```python
from build123d import *

# Parameters (mm, degrees)
F0_W     = 977.9
F0_H     = 38.1
F1_DEPTH = 19.05
F3_DEPTH = 25.4
F5_DEPTH = 25.4


with BuildPart() as f1:
    # F0 (on Front) → F1 (new body)
    with BuildSketch(Plane.XZ):
        with Locations((-488.95, 19.05)):
            Rectangle(F0_W, F0_H)
    extrude(amount=F1_DEPTH)

    # F2 (on face) → F3 (cut)
    with BuildSketch(Plane.XZ.offset(19.05)):
        Polygon((-971.181942, 0), (-977.9, 38.1), (-977.9, 0), align=None)
    extrude(amount=-F3_DEPTH, mode=Mode.SUBTRACT)

    # F4 (on face) → F5 (cut)
    with BuildSketch(Plane.XZ.offset(19.05)):
        Polygon((0, 0), (0, 38.1), (-6.718058, 0), align=None)
    extrude(amount=-F5_DEPTH, mode=Mode.SUBTRACT)


solid = f1.part
```
Geometry check sheet. Reference: the model listing, model coordinates, mm. Give positions to 0.01 mm unless a question says otherwise; leave off trailing zeros. Answer as CSV lines item,"result".
Item 1: Material ranges on line 1 (X direction, y = -9.5, z = 17); line 2 (X direction, y = -7.5, z = 15.5), recorded low to high.
Values:
line 1,"x = -974.18 to -3.72"
line 2,"x = -973.92 to -3.98"
Item 2: Depth check by flat-ended pin: P1, Ø4, axis at y = -6, z = 12.5, coming from the -X side; P2, Ø3, axis at y = -3.5, z = 12, coming from the -X side. Enter the tip coordinate at first touch or a pass-through.
Values:
P1,"stops at x = -973.74"
P2,"stops at x = -973.56"
Item 3: Release check for a two-part mould opening along Y. For faces 1 (the flat face through (-496, 0, 19)), 2 (the flat face through (-496, -19.05, 19)), 3 (the flat face through (-974.494, -9.658, 18.783)) record: pulls with the +Y half, pulls with the -Y half, needs draft (parallel to the pull), parting line crosses it, or undercut.
Values:
face 1,"pulls with the +Y half"
face 2,"pulls with the -Y half"
face 3,"needs draft"
